```python
from build123d import *

# Parameters (mm, degrees)
CYLINDER_R     = 3
CYLINDER_DEPTH = 10
SKETCH009_W    = 29.3
SKETCH009_H    = 16
PAD010_DEPTH   = 16
SKETCH010_W    = 33.3
SKETCH010_H    = 20
PAD009_DEPTH   = 13


with BuildPart() as zylinder:
    # Cylinder → Cylinder (new body)
    with BuildSketch(Plane(origin=(-83, -21, 10), x_dir=(0, 0, -1), z_dir=(1, 0, 0))):
        Circle(CYLINDER_R)
    extrude(amount=CYLINDER_DEPTH)


with BuildPart() as body_innen:
    # Sketch009 → Pad010 (new body)
    with BuildSketch(Plane.XY):
        Rectangle(SKETCH009_W, SKETCH009_H)
    extrude(amount=PAD010_DEPTH)


with BuildPart() as cut006:
    # Sketch010 → Pad009 (new body)
    with BuildSketch(Plane.XY):
        Rectangle(SKETCH010_W, SKETCH010_H)
    extrude(amount=PAD009_DEPTH)

    # Cut005: cut Body innen
    add(body_innen.part, mode=Mode.SUBTRACT)


with BuildPart() as cut006_1:
    # Cut005 placement: moved
    add(cut006.part.moved(Location((-63, -21, 3))))

    # Cut006: cut Zylinder
    add(zylinder.part, mode=Mode.SUBTRACT)


with BuildPart() as cut006_2:
    # Cut006 placement: moved
    add(cut006_1.part.moved(Location((0, 38, 0))))


solid = cut006_2.part
```
Work out the finished part from the listing and answer in its coordinate system (mm). A direction names the side the tool comes from. Coordinates: 2 decimals unless noted, no trailing zeros. Order: outer loops, then holes, each group sorted by start corner. A loop starts at its lowest first (then second) coordinate and runs counter-clockwise, first axis right, second up. Notation, with made-up numbers: (-10, 64) - (47, 64) arc R28 cw to (47, 91) - close; hole circle Ø5 at (61, 18). An arc over 180 degrees is marked (long way). Answer as a JSON object with one key per item and string values.
1. Find section B-B on y = 17. Determine the outline of the cut face in (x, z), plus the area to 3 significant figures.
Output values:
{"outline": "(-79.65, 3) - (-77.65, 3) - (-77.65, 7) - (-79.65, 7) - close; (-79.65, 13) - (-77.65, 13) - (-77.65, 16) - (-79.65, 16) - close; (-48.35, 3) - (-46.35, 3) - (-46.35, 16) - (-48.35, 16) - close", "area": "40.0 mm²"}
2. A tool of negligible diameter and unlimited length cuts with its end or side. For faces 1 (the face through (-63, 9, 9)), 2 (the face through (-63.1, 25.2, 16)), from which of +Z, -Z, +X, -X, +Y, -Y can it reach the whole face along a straight path? Write none if from no direction.
Output values:
{"face 1": "+Z, -Z", "face 2": "+Z, +X, -X, +Y, -Y"}
3. This flat-tipped pin is pushed along its axis until it touches: P1, Ø4, axis at x = -50.5, y = 15, coming from the -Z side. Where does it stop, or does it pass through?
Output values:
{"P1": "passes through"}
4. The mould has two halves that part along X. Classify faces 3 (the face through (-63, 25, 9)), 4 (the face through (-79.65, 16.9, 6.5)), 5 (the face through (-78.66, 14.07, 10.65)): +X half, -X half, draft (parallel to the pull), parting line (faces both ways), or undercut.
Output values:
{"face 3": "undercut", "face 4": "-X half", "face 5": "draft"}
5. Find section A-A on y = 23.5. Determine the outline of the cut face in (x, z).
Output values:
{"outline": "(-79.65, 3) - (-77.65, 3) - (-77.65, 16) - (-79.65, 16) - close; (-48.35, 3) - (-46.35, 3) - (-46.35, 16) - (-48.35, 16) - close"}
6. Find section C-C on x = -71. Determine the outline of the cut face in (y, z), plus the area to 3 significant figures.
Output values:
{"outline": "(7, 3) - (9, 3) - (9, 16) - (7, 16) - close; (25, 3) - (27, 3) - (27, 16) - (25, 16) - close", "area": "52.0 mm²"}
7. Consider line 1 (X direction, y = 17, z = 4.75); line 2 (Z direction, x = -78.45, y = 17); line 3 (Y direction, x = -58, z = 10.75). Determine where each line is inside the solid, lowest interval first.
Output values:
{"line 1": "x = -79.65 to -77.65, -48.35 to -46.35", "line 2": "z = 3 to 7, 13 to 16", "line 3": "y = 7 to 9, 25 to 27"}
8. Find section D-D on z = 10. Determine the outline of the cut face in (x, y), plus the area to 3 significant figures.
Output values:
{"outline": "(-79.65, 7) - (-46.35, 7) - (-46.35, 27) - (-79.65, 27) - (-79.65, 20) - (-77.65, 20) - (-77.65, 25) - (-48.35, 25) - (-48.35, 9) - (-77.65, 9) - (-77.65, 14) - (-79.65, 14) - close", "area": "185 mm²"}
